Verification items for the finished model (mm, model axes). A direction names the side the tool comes from. Give positions to 0.01 mm unless a question says otherwise; leave off trailing zeros. Write each loop counter-clockwise with the first axis right and the second up, starting at its lowest first coordinate (ties: lowest second). Pieces come first, ordered by that corner, then holes.
from build123d import *


with BuildPart() as part:
    # Sketch1 → Revolve1 (revolve)
    with BuildSketch(Plane.XY, mode=Mode.PRIVATE) as revolve1_sk:
        with BuildLine():
            Line((5.628277432, 36.754630752), (7.372072988, 36.754630752))
            Line((7.372072988, 36.754630752), (8.226027868, 35.274630752))
            Line((8.226027868, 35.274630752), (8.826027868, 35.274630752))
            Line((8.826027868, 35.274630752), (9.826027868, 34.274630752))
            Line((9.826027868, 34.274630752), (9.826027868, 22.274630752))
            Line((9.826027868, 22.274630752), (8.826027868, 21.274630752))
            Line((8.826027868, 21.274630752), (4.826027868, 21.274630752))
            ThreePointArc((4.826027868, 21.274630752), (4.118921087, 20.981737533), (3.826027868, 20.274630752))
            Line((3.826027868, 20.274630752), (3.826027868, 5.174630752))
            Line((3.826027868, 5.174630752), (-0.173972132, 5.174630752))
            Line((-0.173972132, 5.174630752), (-0.173972132, 40.524630752))
            ThreePointArc((-0.173972132, 40.524630752), (3.285760517, 39.499360792), (5.628277432, 36.754630752))
        make_face()
    revolve(revolve1_sk.sketch.rotate(Axis((-0.173972132, 0, 0), (0, 1, 0)), 90), axis=Axis((-0.173972132, 0, 0), (0, 1, 0)))


solid = part.part
Item 1: Scan lines: line 1 along Y through (x, z) = (7.25, -0.5); line 2 along Y through (x, z) = (2, -8.5); line 3 along X through (y, z) = (26.5, 1.5). Record each from-to range of solid material in increasing order.
Answer key:
line 1: y = 21.27 to 36.75
line 2: y = 21.27 to 35.27
line 3: x = -10.06 to 9.71
Item 2: Set-up check for faces 1 (the face through (-0.61, 28.19, 9.99)), 2 (the face through (4, 21.275, -4)), 3 (the face through (5.4, 36.755, 2.2)): record each of +Z, -Z, +X, -X, +Y, -Y from which the full face is reachable in a straight line by a thin tool's end or side.
Answer key:
face 1: +Y, -Y
face 2: -Y
face 3: +Y
Item 3: Sectioned sample at B-B on y = 37.5. Record the cut outline in (x, z).
Answer key:
outline: circle Ø10.82 at (-0.17, 0)
Item 4: Sectioned sample at C-C on y = 24. Record the cut outline in (x, z).
Answer key:
outline: circle Ø20 at (-0.17, 0)
Item 5: Depth check by flat-ended pin: pin 1 (8 mm diameter, centred on x = 7, z = -3, fed in from +Y); pin 2 (6 mm diameter, centred on x = 0, y = 9, fed in from -Z); pin 3 (5 mm diameter, centred on x = 2, y = 19, fed in from +Z); pin 4 (1 mm diameter, centred on x = 5.5, y = 13, fed in from -Z). Enter the tip coordinate at first touch or a pass-through.
Answer key:
pin 1: stops at y = 39.28
pin 2: stops at z = -4
pin 3: stops at z = 9.02
pin 4: passes through
Item 6: Sectioned sample at A-A on z = 0. Record the cut outline in (x, y), then the cut area to 3 significant figures.
Answer key:
outline: (-10.17, 22.27) - (-9.17, 21.27) - (-5.17, 21.27) arc R1 cw to (-4.17, 20.27) - (-4.17, 5.17) - (3.83, 5.17) - (3.83, 20.27) arc R1 cw to (4.83, 21.27) - (8.83, 21.27) - (9.83, 22.27) - (9.83, 34.27) - (8.83, 35.27) - (8.23, 35.27) - (7.37, 36.75) - (5.63, 36.75) arc R6.35 ccw to (-5.98, 36.75) - (-7.72, 36.75) - (-8.57, 35.27) - (-9.17, 35.27) - (-10.17, 34.27) - close
area: 462 mm2
